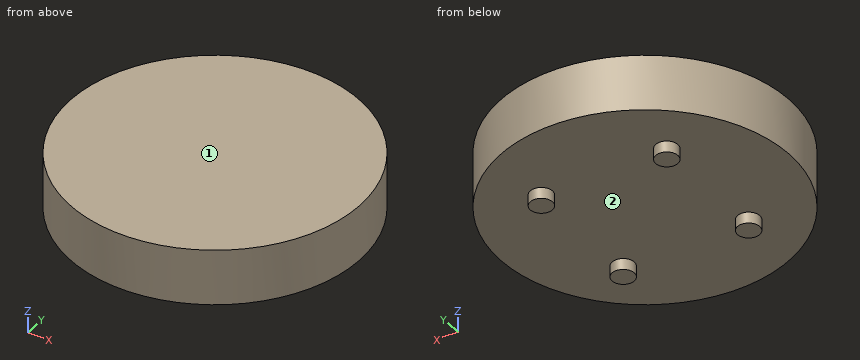
from build123d import *

# Parameters (mm, degrees)
SKETCH_1_R      = 130
EXTRUDE_1_DEPTH = 50
SKETCH_4_R      = 10
EXTRUDE_4_DEPTH = 10


with BuildPart() as part:
    # 草图1 → 凸台-拉伸1 (new body)
    with BuildSketch(Plane.XY):
        Circle(SKETCH_1_R)
    extrude(amount=EXTRUDE_1_DEPTH)

    # 草图4 → 凸台-拉伸4 (add)
    with BuildSketch(Plane(origin=(0, 0, 0), x_dir=(-1, 0, 0), z_dir=(0, 0, -1))):
        with Locations(Location((-56.568542495, 56.568542495, 0), (0, 0, 180))):
            Circle(SKETCH_4_R)
        with Locations(Location((56.568542495, 56.568542495, 0), (0, 0, 180))):
            Circle(SKETCH_4_R)
        with Locations(Location((-56.568542495, -56.568542495, 0), (0, 0, 180))):
            Circle(SKETCH_4_R)
        with Locations(Location((56.568542495, -56.568542495, 0), (0, 0, 180))):
            Circle(SKETCH_4_R)
    extrude(amount=EXTRUDE_4_DEPTH)


solid = part.part
The listing builds one solid part. Answer for the finished solid, in the listing's coordinates (mm). Face numbers are marked on the shaded views. A direction names the side the tool comes from. Give positions to 0.01 mm unless a question says otherwise; leave off trailing zeros. Loops run counter-clockwise (first coordinate to the right, second up) from the corner with the lowest first, then second, coordinate; pieces in that order, holes last. Notation, with made-up numbers: (81, 64) - (130, 64) arc R22 cw to (130, 92) - close; hole circle Ø1 at (70.25, -9.5). An arc over 180 degrees is marked (long way). Answer as a JSON object with one key per item and string values.
1. Find the intervals of material crossed by L1, parallel to X at y = -2, z = 41; L2, parallel to Z at x = 109, y = 23; L3, parallel to Y at x = -0.5, z = 33.5, in increasing order. Write a range as [from, to].
Determined:
{"L1": "[-129.98, 129.98]", "L2": "[0, 50]", "L3": "[-130, 130]"}
2. A cutting plane is placed at C-C (z = 27). Write down the section's boundary in (x, y), then the cut area to 3 significant figures.
Determined:
{"outline": "circle Ø260 at (0, 0)", "area": "53,100 mm²"}
3. A cutting plane is placed at A-A (x = 0). Write down the section's boundary in (y, z), then the cut area to 3 significant figures.
Determined:
{"outline": "(-130, 0) - (130, 0) - (130, 50) - (-130, 50) - close", "area": "13,000 mm²"}
4. Flat-ended cylindrical pins translate along their axes: pin 1 Ø5 at (x, z) = (48, 22) entering from -Y; pin 2 Ø3 at (y, z) = (-55, 3.5) entering from +X; pin 3 Ø2 at (y, z) = (42.5, 39) entering from +X. Find the tip coordinate at first contact, or state that the pin passes through.
Determined:
{"pin 1": "y = -121.78", "pin 2": "x = 118.48", "pin 3": "x = 123.2"}
5. For the marked faces 1 and 2, determine the directions among +Z, -Z, +X, -X, +Y, -Y from which every point of the face is accessible in a straight line to the end or side of a thin tool.
Determined:
{"face 1": "+Z, +X, -X, +Y, -Y", "face 2": "-Z"}
